Could you check a few things on this model? Use its own coordinates, in mm. Give positions to 0.01 mm unless a question says otherwise; leave off trailing zeros. Loops run counter-clockwise (first coordinate to the right, second up) from the corner with the lowest first, then second, coordinate; pieces in that order, holes last.
1. For P1, Ø6.5, axis at x = 355, y = 20, coming from the +Z side; P2, Ø4, axis at x = 9, z = 8, coming from the -Y side; P3, Ø3.5, axis at x = 353.5, y = 68, coming from the -Z side, each with a flat end and sliding along its axis, tell me the tip position at first contact or that it passes through.
2. I need wall thicknesses on line 1 along Y through (x, z) = (355, 8.75); line 2 along Y through (x, z) = (371, 10.75); line 3 along Z through (x, y) = (44, 6.75). Which ranges of each line are inside material? Lowest first, please.
3. Imagine slicing it at A-A (x = 355). List the corners of the cut face in (y, z) for me.
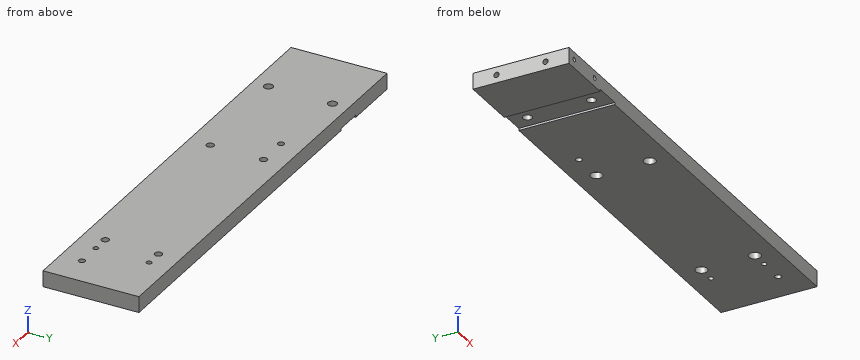
```python
from build123d import *

# Parameters (mm, degrees)
SKETCH_1_W                     = 425
SKETCH_1_H                     = 90
EXTRUDE_1_DEPTH                = 15
SKETCH_2_W                     = 25
SKETCH_2_H                     = 2
CUT_EXTRUDE_1_DEPTH            = 435.683793119
HOLE_WIZARD_M10_1_D            = 8.5
HOLE_WIZARD_M10_1_DEPTH        = 24.5
HOLE_WIZARD_M10_1_TIP          = 2.553657631
HOLE_WIZARD_M6_1_D             = 5
HOLE_WIZARD_M6_1_DEPTH         = 15
HOLE_WIZARD_M6_1_TIP           = 1.502151548
HOLE_WIZARD_M5_1_D             = 4.2
HOLE_WIZARD_M5_1_DEPTH         = 12.4
HOLE_WIZARD_M5_1_TIP           = 1.2618073
HOLE_WIZARD_M6_2_D             = 5
HOLE_WIZARD_M6_2_DEPTH         = 15
HOLE_WIZARD_M6_2_TIP           = 1.502151548
SKETCH_11_R                    = 3
CUT_EXTRUDE_2_DEPTH            = 435.683793119
HOLE_WIZARD_M6_1_2_D           = 7
HOLE_WIZARD_M6_1_2_CBORE_D     = 11
HOLE_WIZARD_M6_1_2_CBORE_DEPTH = 6


with BuildPart() as part:
    # 草图1 → 凸台-拉伸1 (new body)
    with BuildSketch(Plane.XY):
        with Locations((212.5, 45)):
            Rectangle(SKETCH_1_W, SKETCH_1_H)
    extrude(amount=EXTRUDE_1_DEPTH)

    # 草图2 → 切除-拉伸1 (cut, through all)
    with BuildSketch(Plane(origin=(0, 90, 0), x_dir=(1, 0, 0), z_dir=(0, 1, 0))):
        with Locations((66, -1)):
            Rectangle(SKETCH_2_W, SKETCH_2_H)
    extrude(amount=-CUT_EXTRUDE_1_DEPTH, mode=Mode.SUBTRACT)

    # M10 螺纹孔1
    with Locations(Plane(origin=(0, 0, 2), x_dir=(-1, 0, 0), z_dir=(0, 0, -1))):
        with Locations((-66, 75), (-66, 15)):
            Hole(HOLE_WIZARD_M10_1_D / 2, depth=HOLE_WIZARD_M10_1_DEPTH)
            with Locations((0, 0, -(HOLE_WIZARD_M10_1_DEPTH + HOLE_WIZARD_M10_1_TIP / 2))):  # 118° drill point
                Cone(0, HOLE_WIZARD_M10_1_D / 2, HOLE_WIZARD_M10_1_TIP, mode=Mode.SUBTRACT)

    # Hole Wizard M6 _1
    with Locations(Plane.ZY):
        with Locations((7.5, 68), (7.5, 22)):
            Hole(HOLE_WIZARD_M6_1_D / 2, depth=HOLE_WIZARD_M6_1_DEPTH)
            with Locations((0, 0, -(HOLE_WIZARD_M6_1_DEPTH + HOLE_WIZARD_M6_1_TIP / 2))):  # 118° drill point
                Cone(0, HOLE_WIZARD_M6_1_D / 2, HOLE_WIZARD_M6_1_TIP, mode=Mode.SUBTRACT)

    # M5 螺纹孔1
    with Locations(Plane.XZ):
        with Locations((9, 8), (44, 8)):
            Hole(HOLE_WIZARD_M5_1_D / 2, depth=HOLE_WIZARD_M5_1_DEPTH)
            with Locations((0, 0, -(HOLE_WIZARD_M5_1_DEPTH + HOLE_WIZARD_M5_1_TIP / 2))):  # 118° drill point
                Cone(0, HOLE_WIZARD_M5_1_D / 2, HOLE_WIZARD_M5_1_TIP, mode=Mode.SUBTRACT)

    # M6 螺纹孔2
    with Locations(Plane(origin=(0, 0, 0), x_dir=(-1, 0, 0), z_dir=(0, 0, -1))):
        with Locations((-371, 70), (-371, 20)):
            Hole(HOLE_WIZARD_M6_2_D / 2, depth=HOLE_WIZARD_M6_2_DEPTH)
            with Locations((0, 0, -(HOLE_WIZARD_M6_2_DEPTH + HOLE_WIZARD_M6_2_TIP / 2))):  # 118° drill point
                Cone(0, HOLE_WIZARD_M6_2_D / 2, HOLE_WIZARD_M6_2_TIP, mode=Mode.SUBTRACT)

    # 草图11 → 切除-拉伸2 (cut, through all)
    with BuildSketch(Plane(origin=(0, 0, 0), x_dir=(-1, 0, 0), z_dir=(0, 0, -1))):
        with Locations((-145, 70)):
            Circle(SKETCH_11_R)
        with Locations((-395, 20)):
            Circle(SKETCH_11_R)
    extrude(amount=-CUT_EXTRUDE_2_DEPTH, mode=Mode.SUBTRACT)

    # Hole Wizard M6 _1 2 (through all)
    with Locations(Plane(origin=(0, 0, 0), x_dir=(-1, 0, 0), z_dir=(0, 0, -1))):
        with Locations((-175, 20), (-355, 20), (-175, 70), (-355, 70)):
            CounterBoreHole(HOLE_WIZARD_M6_1_2_D / 2, HOLE_WIZARD_M6_1_2_CBORE_D / 2, HOLE_WIZARD_M6_1_2_CBORE_DEPTH)


solid = part.part
```
Derived:
1. P1: passes through
1. P2: stops at y = 12.46
1. P3: stops at z = 6
2. line 1: y = 0 to 16.5, 23.5 to 66.5, 73.5 to 90
2. line 2: y = 0 to 17.5, 22.5 to 67.5, 72.5 to 90
2. line 3: z = 0 to 5.9, 10.1 to 15
3. outline: (0, 0) - (14.5, 0) - (14.5, 6) - (16.5, 6) - (16.5, 15) - (0, 15) - close; (23.5, 6) - (25.5, 6) - (25.5, 0) - (64.5, 0) - (64.5, 6) - (66.5, 6) - (66.5, 15) - (23.5, 15) - close; (73.5, 6) - (75.5, 6) - (75.5, 0) - (90, 0) - (90, 15) - (73.5, 15) - close
